```python
from build123d import *

# Parameters (mm, degrees)
F0_R     = 2.2
F1_DEPTH = 4
F2_R     = 3
F2_R_2   = 1.5
F3_DEPTH = 6


with BuildPart() as f1:
    # F0 (on Top) → F1 (new body)
    with BuildSketch(Plane.XY):
        with BuildLine():
            ThreePointArc((47.5, 32), (46.328427, 34.828427), (43.5, 36))
            Line((43.5, 36), (-43.5, 36))
            ThreePointArc((-43.5, 36), (-46.328427, 34.828427), (-47.5, 32))
            Line((-47.5, 32), (-47.5, 24))
            ThreePointArc((-47.5, 24), (-46.328427, 21.171573), (-43.5, 20))
            Line((-43.5, 20), (-14, 20))
            ThreePointArc((-14, 20), (-11.171573, 18.828427), (-10, 16))
            Line((-10, 16), (-10, -16))
            ThreePointArc((-10, -16), (-11.171573, -18.828427), (-14, -20))
            Line((-14, -20), (-43.5, -20))
            ThreePointArc((-43.5, -20), (-46.328427, -21.171573), (-47.5, -24))
            Line((-47.5, -24), (-47.5, -32))
            ThreePointArc((-47.5, -32), (-46.328427, -34.828427), (-43.5, -36))
            Line((-43.5, -36), (43.5, -36))
            ThreePointArc((43.5, -36), (46.328427, -34.828427), (47.5, -32))
            Line((47.5, -32), (47.5, -24))
            ThreePointArc((47.5, -24), (46.328427, -21.171573), (43.5, -20))
            Line((43.5, -20), (14, -20))
            ThreePointArc((14, -20), (11.171573, -18.828427), (10, -16))
            Line((10, -16), (10, 16))
            ThreePointArc((10, 16), (11.171573, 18.828427), (14, 20))
            Line((14, 20), (43.5, 20))
            ThreePointArc((43.5, 20), (46.328427, 21.171573), (47.5, 24))
            Line((47.5, 24), (47.5, 32))
        make_face()
        Circle(F0_R, mode=Mode.SUBTRACT)
    extrude(amount=F1_DEPTH)

    # F2 (on face) → F3 (join)
    with BuildSketch(Plane.XY.offset(4)):
        with Locations((-42.5, 31)):
            Circle(F2_R)
        with Locations((-42.5, 31)):
            Circle(F2_R_2, mode=Mode.SUBTRACT)
        with Locations((42.5, 31)):
            Circle(F2_R)
        with Locations((42.5, 31)):
            Circle(F2_R_2, mode=Mode.SUBTRACT)
        with Locations((42.5, -31)):
            Circle(F2_R)
        with Locations((42.5, -31)):
            Circle(F2_R_2, mode=Mode.SUBTRACT)
        with Locations((-42.5, -31)):
            Circle(F2_R)
        with Locations((-42.5, -31)):
            Circle(F2_R_2, mode=Mode.SUBTRACT)
    extrude(amount=F3_DEPTH)


solid = f1.part
```
The model under review builds one solid part; all positions refer to its coordinate system, in mm. A direction names the side the tool comes from. Round coordinates to 2 decimals unless told otherwise and drop trailing zeros. Order: outer loops, then holes, each group sorted by start corner. A loop starts at its lowest first (then second) coordinate and runs counter-clockwise, first axis right, second up. Notation, with made-up numbers: (66.25, 66) -> (92.25, 66) arc R25 cw to (92.25, 97) -> close; hole circle Ø9 at (-29, 80). An arc over 180 degrees is marked (long way). One line per item, written item: value. Start each with the question number.
Q1. Wall thickness on line 1 (Y direction, x = -42.5, z = 7.75); line 2 (Z direction, x = -6, y = -27.5); line 3 (Y direction, x = 40.5, z = 1): over which ranges is each line inside the solid? List them lowest first.
Q2. Take a section at A-A (z = 5.75). Write out the cut boundary in (x, y), and give its area (3 significant figures).
Q3. Mouldability with a two-part tool opening along X and no side actions: class faces 5 (the face through (-10, 0, 2)), 6 (the face through (-1, 9, 4)), 7 (the face through (11.141, 18.797, 1.972)) as released by +X, released by -X, zero draft, split by the parting line, or undercut.
Q4. Machinability: for faces 1 (the face through (-43, -31, 4)), 2 (the face through (46.297, 21.141, 1.972)), 3 (the face through (47.5, 28, 2)), 4 (the face through (-29, 20, 2)), which of the approach directions +Z, -Z, +X, -X, +Y, -Y give a long, thin tool a straight path to every point of the face, cutting with its end or side? Answer none if there is none.
Q5. Take a section at D-D (x = 42.5). Write out the cut boundary in (y, z).
Q6. Take a section at B-B (x = 0). Write out the cut boundary in (y, z), and give its area (3 significant figures).
Q7. Clearance check with flat-ended pins moving along their axes: pin 1 Ø3.5 at (x, y) = (42.5, -31) entering from +Z; pin 2 Ø4 at (y, z) = (20.5, 2) entering from +X; pin 3 Ø0.9 at (x, y) = (43, 31.5) entering from +Z; pin 4 Ø4.5 at (y, z) = (-2.5, 3) entering from -X. State where each tip first meets the part, or that it passes through.
Q8. Take a section at C-C (y = 0). Write out the cut boundary in (x, z), and give its area (3 significant figures).
Reported:
1. line 1: y = -34 to -32.5, -29.5 to -28, 28 to 29.5, 32.5 to 34
1. line 2: z = 0 to 4
1. line 3: y = -36 to -20, 20 to 36
2. outline: circle Ø6 at (-42.5, -31); circle Ø6 at (-42.5, 31); circle Ø6 at (42.5, -31); circle Ø6 at (42.5, 31); hole circle Ø3 at (-42.5, -31); hole circle Ø3 at (-42.5, 31); hole circle Ø3 at (42.5, -31); hole circle Ø3 at (42.5, 31)
2. area: 84.8 mm2
3. face 5: released by -X
3. face 6: undercut
3. face 7: released by +X
4. face 1: +Z
4. face 2: +Z, -Z, +X
4. face 3: +Z, -Z, +X, +Y, -Y
4. face 4: +Z, -Z, -X
5. outline: (-36, 0) -> (-20, 0) -> (-20, 4) -> (-28, 4) -> (-28, 10) -> (-29.5, 10) -> (-29.5, 4) -> (-32.5, 4) -> (-32.5, 10) -> (-34, 10) -> (-34, 4) -> (-36, 4) -> close; (20, 0) -> (36, 0) -> (36, 4) -> (34, 4) -> (34, 10) -> (32.5, 10) -> (32.5, 4) -> (29.5, 4) -> (29.5, 10) -> (28, 10) -> (28, 4) -> (20, 4) -> close
6. outline: (-36, 0) -> (-2.2, 0) -> (-2.2, 4) -> (-36, 4) -> close; (2.2, 0) -> (36, 0) -> (36, 4) -> (2.2, 4) -> close
6. area: 270 mm2
7. pin 1: stops at z = 10
7. pin 2: stops at x = 47.21
7. pin 3: stops at z = 4
7. pin 4: stops at x = -10
8. outline: (-10, 0) -> (-2.2, 0) -> (-2.2, 4) -> (-10, 4) -> close; (2.2, 0) -> (10, 0) -> (10, 4) -> (2.2, 4) -> close
8. area: 62.4 mm2
